from build123d import *

# Parameters (mm, degrees)
BOSS_EXTRUDE1_DEPTH = 706
FILLET1_R           = 1.5
CUT_EXTRUDE1_DEPTH  = 708.733000502
CUT_EXTRUDE2_DEPTH  = 10
FILLET2_R           = 4
FILLET3_R           = 4
FILLET4_R           = 4
FILLET5_R           = 4
CUT_EXTRUDE3_DEPTH  = 10


with BuildPart() as part:
    # Sketch1 → Boss-Extrude1 (new, symmetric)
    with BuildSketch(Plane.XY):
        with BuildLine():
            Line((-1, 0), (-35, 0))
            Line((-35, 0), (-35, 3))
            Line((-35, 3), (-6, 3))
            ThreePointArc((-6, 3), (-3.878679656, 3.878679656), (-3, 6))
            Line((-3, 6), (-3, 35))
            Line((-3, 35), (0, 35))
            Line((0, 35), (0, 1))
            ThreePointArc((0, 1), (-0.292893219, 0.292893219), (-1, 0))
        make_face()
    extrude(amount=BOSS_EXTRUDE1_DEPTH, both=True)

    # Fillet1
    fillet1_edges = [part.edges().sort_by_distance(p)[0] for p in [
        (-35, 3, 0),
        (-3, 35, 0),
    ]]
    fillet(fillet1_edges, radius=FILLET1_R)

    # Sketch2 → Cut-Extrude1 (cut, through all)
    with BuildSketch(Plane.XZ):
        Polygon((-35, -706), (0, -671), (0, -706), align=None)
    cut_extrude1 = extrude(amount=-CUT_EXTRUDE1_DEPTH, mode=Mode.SUBTRACT)

    # Sketch3 → Cut-Extrude2 (cut)
    with BuildSketch(Plane(origin=(0, 0, 0), x_dir=(0, 0, -1), z_dir=(1, 0, 0))):
        Polygon((642, 35), (674, 3), (706, 3), (674, 35), align=None)
    cut_extrude2 = extrude(amount=-CUT_EXTRUDE2_DEPTH, mode=Mode.SUBTRACT)

    # Mirror1: Cut-Extrude1, Cut-Extrude2 across plane
    add(cut_extrude1.mirror(Plane.XY), mode=Mode.SUBTRACT)
    add(cut_extrude2.mirror(Plane.XY), mode=Mode.SUBTRACT)

    # Fillet2
    # the kernel refuses this fillet: 4 mm, written as the material it takes off along each edge
    with BuildSketch(Plane(origin=(4.142135624, 35, -642), x_dir=(0, 0, 1), z_dir=(-1, 0, 0))) as fillet2_piece_1:
        with BuildLine():
            CenterArc((FILLET2_R * 0.414213562373, -FILLET2_R), FILLET2_R, 90, 45)
            Line((-FILLET2_R * 0.292893218813, -FILLET2_R * 0.292893218813), (0, 0))
            Line((0, 0), (FILLET2_R * 0.414213562373, 0))
        make_face()
    extrude(amount=9.784271247, mode=Mode.SUBTRACT)

    # Fillet3
    # the kernel refuses this fillet: 4 mm, written as the material it takes off along each edge
    with BuildSketch(Plane(origin=(0, -3.142135624, -671), x_dir=(-0.707106781186569, 0, -0.707106781186526), z_dir=(0, 1, 0))) as fillet3_piece_1:
        with BuildLine():
            CenterArc((FILLET3_R * 0.414213562373, FILLET3_R), FILLET3_R, 225, 45)
            Line((-FILLET3_R * 0.292893218813, FILLET3_R * 0.292893218813), (0, 0))
            Line((0, 0), (FILLET3_R * 0.414213562373, 0))
        make_face()
    extrude(amount=13.284271247, mode=Mode.SUBTRACT)

    # Fillet4
    # the kernel refuses this fillet: 4 mm, written as the material it takes off along each edge
    with BuildSketch(Plane(origin=(0, -3.142135624, 671), x_dir=(-0.707106781186569, 0, 0.707106781186526), z_dir=(0, 1, 0))) as fillet4_piece_1:
        with BuildLine():
            CenterArc((FILLET4_R * 0.414213562373, -FILLET4_R), FILLET4_R, 90, 45)
            Line((-FILLET4_R * 0.292893218813, -FILLET4_R * 0.292893218813), (0, 0))
            Line((0, 0), (FILLET4_R * 0.414213562373, 0))
        make_face()
    extrude(amount=13.284271247, mode=Mode.SUBTRACT)

    # Fillet5
    # the kernel refuses this fillet: 4 mm, written as the material it takes off along each edge
    with BuildSketch(Plane(origin=(4.142135624, 35, 642), x_dir=(0, -0.7071067811865432, 0.7071067811865518), z_dir=(-1, 0, 0))) as fillet5_piece_1:
        with BuildLine():
            CenterArc((FILLET5_R * 0.414213562373, -FILLET5_R), FILLET5_R, 90, 45)
            Line((-FILLET5_R * 0.292893218813, -FILLET5_R * 0.292893218813), (0, 0))
            Line((0, 0), (FILLET5_R * 0.414213562373, 0))
        make_face()
    extrude(amount=9.784271247, mode=Mode.SUBTRACT)

    # Sketch4 → Cut-Extrude3 (cut)
    with BuildSketch(Plane.ZY.offset(35)):
        Polygon((711.147996861, -1.5), (711.147996861, 1.5), (706, 1.5), (706, 1), (706, 0), (705, 0), (700.876909591, 0), (700.876909591, -1.5), align=None)
        with BuildLine():
            Line((706, 0), (706, 1))
            ThreePointArc((706, 1), (705.707106781, 0.292893219), (705, 0))
            Line((705, 0), (706, 0))
        make_face()
    cut_extrude3 = extrude(amount=-CUT_EXTRUDE3_DEPTH, mode=Mode.SUBTRACT)

    # Mirror2: Cut-Extrude3 across plane
    add(cut_extrude3.mirror(Plane.XY), mode=Mode.SUBTRACT)


solid = part.part
Geometry: final body of the model. Coordinates: model frame, mm. A direction names the side the tool comes from. Coordinates: 2 decimals unless noted, no trailing zeros. Loops run counter-clockwise (first coordinate to the right, second up) from the corner with the lowest first, then second, coordinate; pieces in that order, holes last. Notation, with made-up numbers: M 36,23 L 87,23 A21 cw 87,50 Z; hole C 42.25,-3 d9. An arc over 180 degrees is marked long. One line per item, written item: value. Start each with the question number.
1) Material intervals for L1, parallel to Y at x = -11, z = 242; L2, parallel to X at y = 30, z = -199; L3, parallel to Y at x = -4, z = -75, sorted ascending. Write a range as from..to.
2) Cut plane A-A (z = 493.5). Return loops of the section in (x, y).
3) Pin query (flat end, axial travel): P1, Ø12, axis at y = 12.5, z = 448.5, coming from the -X side. Return the tip coordinate at first contact, or that it passes through.
4) Cut plane B-B (x = -18). Return loops of the section in (y, z).
5) Reachability of faces 1 (the flat face through (-18, 3, 10)), 2 (the flat face through (-18, 0, 10)) from +Z, -Z, +X, -X, +Y, -Y: full face, straight path, thin tool, end or side. Return the list, or none.
6) Cut plane C-C (y = 17). Return loops of the section in (x, z), then the cut area to 3 significant figures.
Evaluation:
1. L1: 0..3
1. L2: -3..0
1. L3: 0..3.76
2. outline: M -35,0 L -1,0 A1 ccw 0,1 L 0,35 L -1.5,35 A1.5 ccw -3,33.5 L -3,6 A3 cw -6,3 L -33.5,3 A1.5 ccw -35,1.5 Z
3. P1: x = -3
4. outline: M 0,-689 L 3,-689 L 3,689 L 0,689 Z
5. face 1: +Z, -Z, -X, +Y
5. face 2: +Z, -Z, +X, -X, -Y
6. outline: M -3,-660 L 0,-660 L 0,660 L -3,660 Z
6. area: 3,960 mm^2
